For this review, take the finished solid that the model builds, in its own axes (mm). A direction names the side the tool comes from. Round coordinates to 2 decimals unless told otherwise and drop trailing zeros. Loops run counter-clockwise (first coordinate to the right, second up) from the corner with the lowest first, then second, coordinate; pieces in that order, holes last.
1. Consider section D-D on y = -23. State the section outline as (x, z) points.
2. Consider section B-B on z = -10. State the section outline as (x, y) points.
3. To check wall thickness, follow line 1 along X through (y, z) = (-20, -10); line 2 along Z through (x, y) = (20, -5.75); line 3 along Z through (x, y) = (-20, -16). State the ranges of each line that lie inside material, in increasing order.
4. Consider section A-A on y = -6. State how many separate pieces and enclosed holes the cut face has, then the cut area to 3 significant figures.
5. Draft analysis for pull direction X (two halves, no side actions). For faces 3 (the cylindrical face through (-29, -2, -3)), 4 (the cylindrical face through (-0.867, -14.79, -13.905)), 5 (the cylindrical face through (28.5, -8.96, 12.07)), state which applies: released by +X, released by -X, zero draft, split by the parting line, or undercut.
6. Tool access review of faces 1 (the flat face through (-30, -15, -6)), 2 (the flat face through (0, -5, 4)): name each direction out of +Z, -Z, +X, -X, +Y, -Y from which nothing blocks a thin tool from reaching the whole face with its end or side.
7. Clearance check with flat-ended pins moving along their axes: pin 1 Ø10.5 at (x, z) = (20, -10) entering from -Y; pin 2 Ø7 at (x, z) = (-9.5, 6) entering from -Y; pin 3 Ø2 at (x, y) = (-8, -23) entering from +Z; pin 4 Ø1.5 at (y, z) = (-18, 1.5) entering from +X. State where each tip first meets the part, or that it passes through.
from build123d import *

# Parameters (mm, degrees)
F0_W     = 60
F0_H     = 20
F1_DEPTH = 30
F2_W     = 60
F2_H     = 8.5
F3_DEPTH = 5
F4_W     = 60
F4_H     = 5
F5_DEPTH = 15
F6_R     = 4
F7_DEPTH = 30.001
F8_R     = 4.99999


# Not quite as in the source:
# - a fillet or chamfer is up to 0.001 mm smaller than in the source, because OpenCascade refuses the exact size


with BuildPart() as f1:
    # F0 (on Front) → F1 (new body)
    with BuildSketch(Plane.XZ):
        with Locations((0, -10)):
            Rectangle(F0_W, F0_H)
    extrude(amount=F1_DEPTH)

    # F2 (on Front) → F3 (join)
    with BuildSketch(Plane.XZ):
        with Locations((0, 4.25)):
            Rectangle(F2_W, F2_H)
    extrude(amount=F3_DEPTH)

    # F4 (on Front) → F5 (join)
    with BuildSketch(Plane.XZ):
        with Locations((0, 11)):
            Rectangle(F4_W, F4_H)
    extrude(amount=F5_DEPTH)

    # F6 (on Front) → F7 (cut, through all)
    with BuildSketch(Plane.XZ):
        with Locations((-20, -10)):
            Circle(F6_R)
        with Locations((0, -10)):
            Circle(F6_R)
        with Locations((20, -10)):
            Circle(F6_R)
    extrude(amount=F7_DEPTH, mode=Mode.SUBTRACT)

    # F8 (radius 5 in the source; OpenCascade refuses exactly that, so slightly less here)
    f8_edges = [f1.edges().sort_by_distance(p)[0] for p in [
        (30, -15, -20),
        (30, -30, -10),
        (30, -7.5, 13.5),
        (0, 0, 13.5),
        (0, 0, -20),
        (-30, -15, -20),
        (0, -30, -20),
        (-30, -30, -10),
        (-30, -7.5, 13.5),
        (-30, 0, -3.25),
        (0, -15, 13.5),
        (30, 0, -3.25),
    ]]
    fillet(f8_edges, radius=F8_R)


solid = f1.part
Resolved:
1. outline: (-30, -15) arc R5 ccw to (-25, -20) - (25, -20) arc R5 ccw to (30, -15) - (30, 0) - (-30, 0) - close; hole circle Ø8 at (-20, -10); hole circle Ø8 at (0, -10); hole circle Ø8 at (20, -10)
2. outline: (-30, -25) arc R5 ccw to (-25, -30) - (-24, -30) - (-24, 0) - (-25, 0) arc R5 ccw to (-30, -5) - close; (-16, -30) - (-4, -30) - (-4, 0) - (-16, 0) - close; (4, -30) - (16, -30) - (16, 0) - (4, 0) - close; (24, -30) - (25, -30) arc R5 ccw to (30, -25) - (30, -5) arc R5 ccw to (25, 0) - (24, 0) - close
3. line 1: x = -30 to -24, -16 to -4, 4 to 16, 24 to 30
3. line 2: z = -20 to -14, -6 to 0, 8.5 to 13.5
3. line 3: z = -20 to -14, -6 to 0
4. separate pieces: 2
4. enclosed holes: 3
4. area: 1,330 mm2
5. face 3: released by -X
5. face 4: undercut
5. face 5: released by +X
6. face 1: +Z, -Z, -X, +Y, -Y
6. face 2: +X, -X, -Y
7. pin 1: stops at y = -30
7. pin 2: stops at y = -15
7. pin 3: stops at z = 0
7. pin 4: passes through
